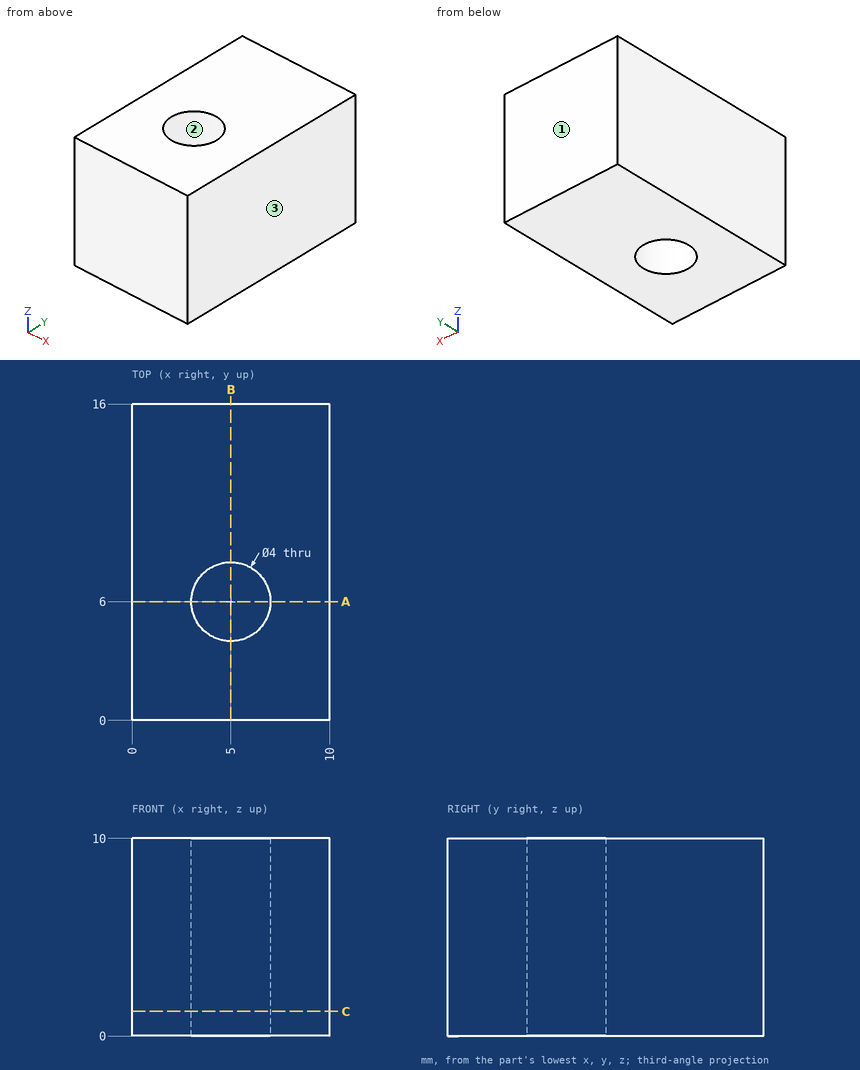
Input: dimensioned drawing with shaded views. Units: mm. Origin: part minimum x, y, z. Give positions to 0.01 mm unless a question says otherwise; leave off trailing zeros. Loops run counter-clockwise (first coordinate to the right, second up) from the corner with the lowest first, then second, coordinate; pieces in that order, holes last. Notation, with made-up numbers: (-23.75, 43) -> (-0.75, 43) arc R11 cw to (-0.75, 60) -> close; hole circle Ø1 at (-25.75, 2.25). An arc over 180 degrees is marked (long way). Return JSON: item names as keys, results as strings.
Item 1: Mould query, pull axis Y, two halves, no side actions, for the marked faces 1, 2 and 3. Classes: released by +Y, released by -Y, zero draft, split by the parting line, or undercut.
Filled in:
{"face 1": "released by +Y", "face 2": "undercut", "face 3": "zero draft"}
Item 2: Section B-B, the plane x = 5. Output: boundary loops of the cut face in (y, z), plus the area to 3 significant figures.
Filled in:
{"outline": "(0, 0) -> (4, 0) -> (4, 10) -> (0, 10) -> close; (8, 0) -> (16, 0) -> (16, 10) -> (8, 10) -> close", "area": "120 mm^2"}
Item 3: Section A-A, the plane y = 6. Output: boundary loops of the cut face in (x, z), plus the area to 3 significant figures.
Filled in:
{"outline": "(0, 0) -> (3, 0) -> (3, 10) -> (0, 10) -> close; (7, 0) -> (10, 0) -> (10, 10) -> (7, 10) -> close", "area": "60.0 mm^2"}
Item 4: Line query: line 1 (Y direction, x = 5, z = 5.75); line 2 (X direction, y = 6.5, z = 4); line 3 (X direction, y = 7.25, z = 4). Output: solid intervals per line, ascending.
Filled in:
{"line 1": "0 to 4, 8 to 16", "line 2": "0 to 3.06, 6.94 to 10", "line 3": "0 to 3.44, 6.56 to 10"}
Item 5: Section C-C, the plane z = 1.25. Output: boundary loops of the cut face in (x, y).
Filled in:
{"outline": "(0, 0) -> (10, 0) -> (10, 16) -> (0, 16) -> close; hole circle Ø4 at (5, 6)"}
